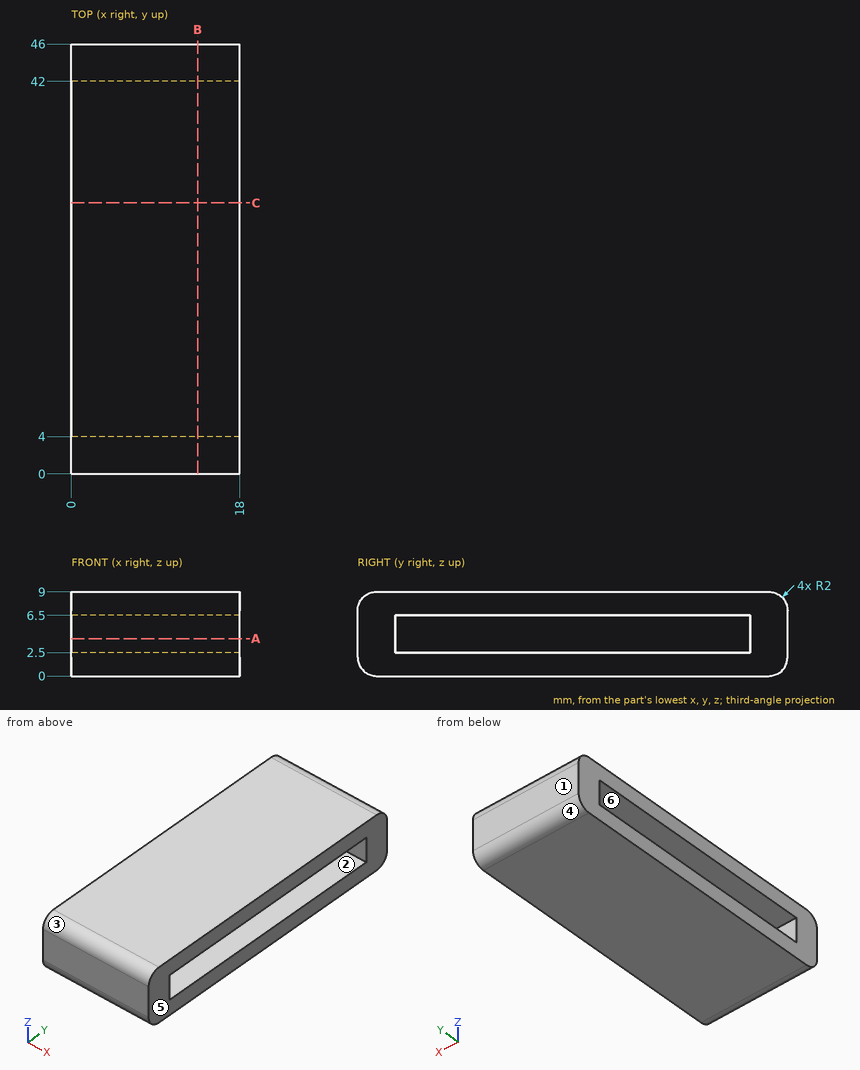
The figure shows three views and two pictorial views of one solid part (mm, origin at its lowest corner). Answer the questions. A direction names the side the tool comes from. Give positions to 0.01 mm unless a question says otherwise; leave off trailing zeros. Loops run counter-clockwise (first coordinate to the right, second up) from the corner with the lowest first, then second, coordinate; pieces in that order, holes last. Notation, with made-up numbers: (35.25, -35) - (73.25, -35) arc R21 cw to (73.25, -9) - close; hole circle Ø5 at (66.5, 83). An arc over 180 degrees is marked (long way). Use one line per item in the form item = value.
1. Section C-C on y = 29 is taken. Give the vertices of the cut face in (x, z), then the cut area to 3 significant figures.
Calculated:
outline = (0, 0) - (18, 0) - (18, 2.5) - (0, 2.5) - close; (0, 6.5) - (18, 6.5) - (18, 9) - (0, 9) - close
area = 90.0 mm^2
2. The mould has two halves that part along Z. Classify the marked faces 3, 4, 5 and 6: pulls with the +Z half, pulls with the -Z half, needs draft (parallel to the pull), parting line crosses it, or undercut.
Calculated:
face_3 = pulls with the +Z half
face_4 = pulls with the -Z half
face_5 = needs draft
face_6 = undercut
3. Find the intervals of material crossed by line 1 along Y through (x, z) = (2.5, 4); line 2 along Z through (x, y) = (11.5, 16); line 3 along Y through (x, z) = (16.75, 1.5), in increasing order. Write a range as [from, to].
Calculated:
line_1 = [0, 4], [42, 46]
line_2 = [0, 2.5], [6.5, 9]
line_3 = [0.06, 45.94]
4. Section A-A on z = 4 is taken. Give the vertices of the cut face in (x, y), then the cut area to 3 significant figures.
Calculated:
outline = (0, 0) - (18, 0) - (18, 4) - (0, 4) - close; (0, 42) - (18, 42) - (18, 46) - (0, 46) - close
area = 144 mm^2
5. Which of the six approach directions +Z, -Z, +X, -X, +Y, -Y give full straight-line access (tool end or side, diameter ignored) to the marked faces 1 and 2?
Calculated:
face_1 = +Z, -Z, +X, -X, +Y
face_2 = +X, -X
6. Section B-B on x = 13.5 is taken. Give the vertices of the cut face in (y, z).
Calculated:
outline = (0, 2) arc R2 ccw to (2, 0) - (44, 0) arc R2 ccw to (46, 2) - (46, 7) arc R2 ccw to (44, 9) - (2, 9) arc R2 ccw to (0, 7) - close; hole (4, 2.5) - (42, 2.5) - (42, 6.5) - (4, 6.5) - close
